Geometry: final body of the model. Coordinates: model frame, mm. Give positions to 0.01 mm unless a question says otherwise; leave off trailing zeros. Order: outer loops, then holes, each group sorted by start corner. A loop starts at its lowest first (then second) coordinate and runs counter-clockwise, first axis right, second up. Notation, with made-up numbers: (47, 17) -> (89, 17) arc R6 ccw to (89, 23) -> close; hole circle Ø9 at (13.5, -35). An arc over 180 degrees is marked (long way). Write item = value, one per line.
```python
from build123d import *

# Parameters (mm, degrees)
SKETCH_W     = 56
SKETCH_H     = 34.8
PAD_DEPTH    = 1.6
SKETCH003_R  = 2
POCKET_DEPTH = 1.601
FILLET_R     = 3


with BuildPart() as part:
    # Sketch → Pad (new body)
    with BuildSketch(Plane.XY):
        Rectangle(SKETCH_W, SKETCH_H)
    extrude(amount=PAD_DEPTH)

    # Sketch003 → Pocket (cut, through all)
    with BuildSketch(Plane.XY.offset(1.6)):
        with Locations((-25.4, -14.5)):
            Circle(SKETCH003_R)
        with Locations((-25.4, 14.5)):
            Circle(SKETCH003_R)
        with Locations((25.4, 14.5)):
            Circle(SKETCH003_R)
        with Locations((25.4, -14.5)):
            Circle(SKETCH003_R)
    extrude(amount=-POCKET_DEPTH, mode=Mode.SUBTRACT)

    # Fillet
    fillet_edges = [part.edges().sort_by_distance(p)[0] for p in [
        (-28, -17.4, 0.8),
        (28, -17.4, 0.8),
        (28, 17.4, 0.8),
        (-28, 17.4, 0.8),
    ]]
    fillet(fillet_edges, radius=FILLET_R)


solid = part.part
```
1) Mould query, pull axis X, two halves, no side actions, for faces 1 (the face through (-23.492, 15.101, 0.811)), 2 (the face through (-27.14, 16.5, 0.81)), 3 (the face through (0, -17.4, 1)). Classes: +X half, -X half, draft (parallel to the pull), parting line (faces both ways), or undercut.
Check sheet entries:
face_1 = undercut
face_2 = -X half
face_3 = draft
2) Section query A-A (z = 0.7). Output: boundary loops of the cut face in (x, y).
Check sheet entries:
outline = (-28, -14.4) arc R3 ccw to (-25, -17.4) -> (25, -17.4) arc R3 ccw to (28, -14.4) -> (28, 14.4) arc R3 ccw to (25, 17.4) -> (-25, 17.4) arc R3 ccw to (-28, 14.4) -> close; hole circle Ø4 at (-25.4, -14.5); hole circle Ø4 at (-25.4, 14.5); hole circle Ø4 at (25.4, -14.5); hole circle Ø4 at (25.4, 14.5)
3) Line query: line 1 (X direction, y = 13.5, z = 0.85); line 2 (Y direction, x = 25.4, z = 0.5); line 3 (Y direction, x = -24, z = 0.5). Output: solid intervals per line, ascending. Write a range as from..to.
Check sheet entries:
line_1 = -28..-27.13, -23.67..23.67, 27.13..28
line_2 = -17.37..-16.5, -12.5..12.5, 16.5..17.37
line_3 = -17.4..-15.93, -13.07..13.07, 15.93..17.4
